Answer from the drawing. Dimensions are ordinates in mm from the lowest x, y and z of the part. A direction names the side the tool comes from. Coordinates: 2 decimals unless noted, no trailing zeros. Write each loop counter-clockwise with the first axis right and the second up, starting at its lowest first coordinate (ties: lowest second). Pieces come first, ordered by that corner, then holes. Notation, with made-up numbers: (29, -38) -> (56, -38) arc R15 cw to (56, -17) -> close; hole circle Ø2 at (-5, 84.5). An arc over 180 degrees is marked (long way). Answer as a JSON object with one key per item and string values. Group by question number.
(1) Find section D-D (y = 10). Give the vertices of the cut face in (x, z).
(2) Straight lines are drawn through the part: L1, parallel to X at y = 2.25, z = 12.5; L2, parallel to Z at x = 12.7, y = 5.5; L3, parallel to X at y = 8.25, z = 12.5. For each, find the intervals that lie inside material, in ascending order.
(3) Find section B-B (x = 12.7). Give the vertices of the cut face in (y, z), then the cut area to 3 significant figures.
(4) Flat-ended cylindrical pins translate along their axes: P1, Ø1, axis at y = 2.5, z = 5, coming from the +X side; P2, Ø4, axis at x = 6, y = 8, coming from the -Z side; P3, Ø1, axis at x = 8, y = 9, coming from the +Z side. Find the tip coordinate at first contact, or state that the pin passes through.
(5) Which of the six approach directions +Z, -Z, +X, -X, +Y, -Y give full straight-line access (tool end or side, diameter ignored) to the marked faces 1 and 2?
(6) Find section A-A (z = 12.7). Give the vertices of the cut face in (x, y).
(7) Find section C-C (x = 3.81). Give the vertices of the cut face in (y, z).
(8) For a pull along X with two mould halves and no side action, classify the marked faces 3, 4 and 5 as +X half, -X half, draft (parallel to the pull), parting line (faces both ways), or undercut.
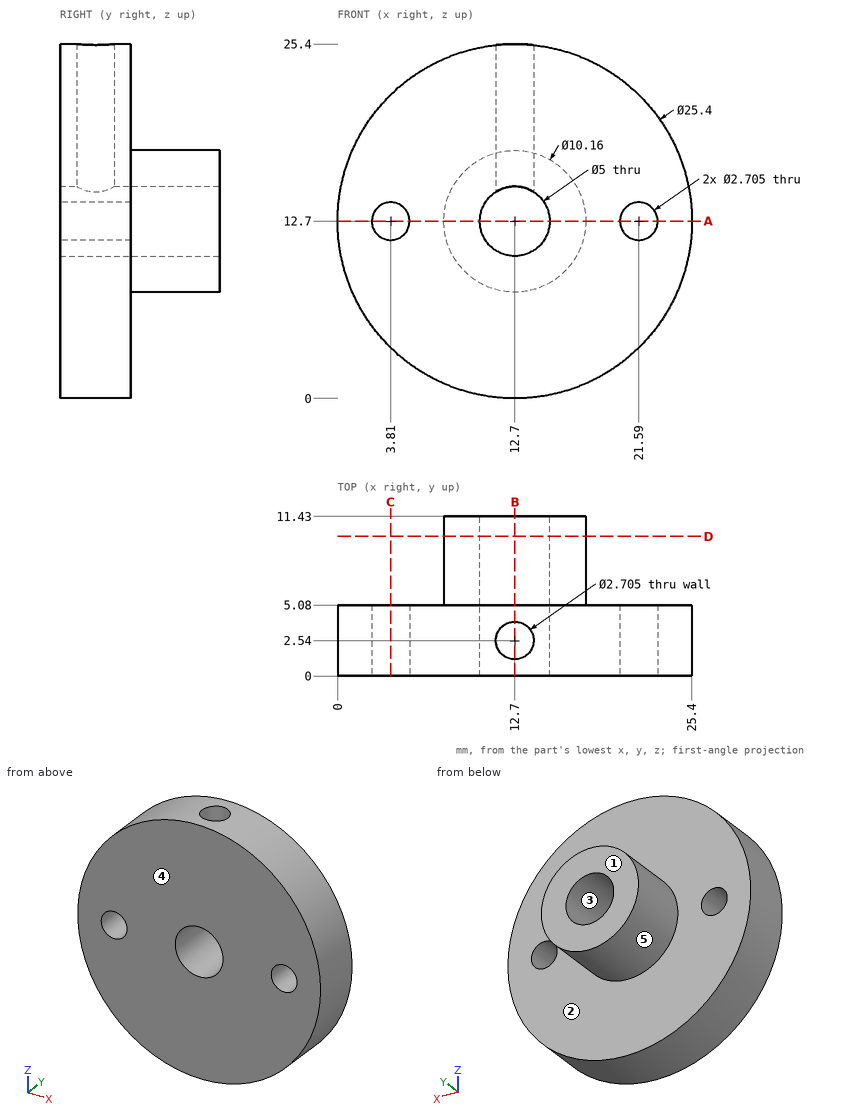
Results below:
{
 "1": {"outline": "circle Ø10.16 at (12.7, 12.7); hole circle Ø5 at (12.7, 12.7)"},
 "2": {"L1": "x = 0 to 2.47, 5.15 to 10.21, 15.19 to 20.25, 22.93 to 25.4", "L2": "z = 7.62 to 10.2, 15.2 to 17.78", "L3": "x = 7.62 to 10.21, 15.19 to 17.78"},
 "3": {"outline": "(0, 0) -> (5.08, 0) -> (5.08, 7.62) -> (11.43, 7.62) -> (11.43, 10.2) -> (0, 10.2) -> close; (0, 15.2) -> (1.19, 15.2) -> (1.19, 25.4) -> (0, 25.4) -> close; (3.89, 15.2) -> (11.43, 15.2) -> (11.43, 17.78) -> (5.08, 17.78) -> (5.08, 25.4) -> (3.89, 25.4) -> close", "area": "109 mm2"},
 "4": {"P1": "stops at x = 23.16", "P2": "stops at z = 10.77", "P3": "stops at z = 15.56"},
 "5": {"face 1": "+Z, -Z, +X, -X, +Y", "face 2": "+Y"},
 "6": {"outline": "(0, 0) -> (2.46, 0) -> (2.46, 5.08) -> (0, 5.08) -> close; (5.16, 0) -> (10.2, 0) -> (10.2, 11.43) -> (7.62, 11.43) -> (7.62, 5.08) -> (5.16, 5.08) -> close; (15.2, 0) -> (20.24, 0) -> (20.24, 5.08) -> (17.78, 5.08) -> (17.78, 11.43) -> (15.2, 11.43) -> close; (22.94, 0) -> (25.4, 0) -> (25.4, 5.08) -> (22.94, 5.08) -> close"},
 "7": {"outline": "(0, 3.63) -> (5.08, 3.63) -> (5.08, 11.35) -> (0, 11.35) -> close; (0, 14.05) -> (5.08, 14.05) -> (5.08, 21.77) -> (0, 21.77) -> close"},
 "8": {"face 3": "undercut", "face 4": "draft", "face 5": "parting line"}
}
